Here's how the part is built. I have some questions about the finished solid (model axes, mm). Face numbers are marked on the shaded views. A direction names the side the tool comes from. Round coordinates to 2 decimals unless told otherwise and drop trailing zeros. Order: outer loops, then holes, each group sorted by start corner. A loop starts at its lowest first (then second) coordinate and runs counter-clockwise, first axis right, second up. Notation, with made-up numbers: (43, -20.75) -> (83, -20.75) arc R30 cw to (83, 17.25) -> close; hole circle Ø6 at (59, 23). An arc over 180 degrees is marked (long way). Use a Markdown table: item, result. Add a question column.
(1) I want a section at A-A, the plane y = 0. Please give me the cut outline in (x, z), then the cut area to 3 significant figures.
(2) If I drill on probe 1 along Y at (x, z) = (14.2, 9); probe 2 along Y at (x, z) = (0, 1); probe 3 along Y at (x, z) = (-5, 5.25), over which ranges is the centre line in solid material (lowest first)?
(3) I want a section at C-C, the plane z = 4.5. Please give me the cut outline in (x, y).
(4) Thinking about a two-plate mould opening in Y: for the marked faces 6, 7 and 8, which applies, pulls with the +Y half, pulls with the -Y half, needs draft (parallel to the pull), parting line crosses it, or undercut?
(5) On a 3-axis mill with a long thin cutter (end or side, diameter ignored), from which of +Z, -Z, +X, -X, +Y, -Y can I reach the whole of each face in a straight line? I mean the marked faces 1, 2, 3, 4 and 5. Say none if no direction works.
(6) I'm going to push flat-ended pins straight in: P1, Ø1.5, axis at x = -14.2, y = -14.2, coming from the +Z side; P2, Ø2, axis at x = -1.5, y = 12, coming from the -Z side; P3, Ø8, axis at x = 5.5, y = -3, coming from the +Z side. Where does each tip first touch, or does it pass through?
(7) I want a section at D-D, the plane y = -6. Please give me the cut outline in (x, z).
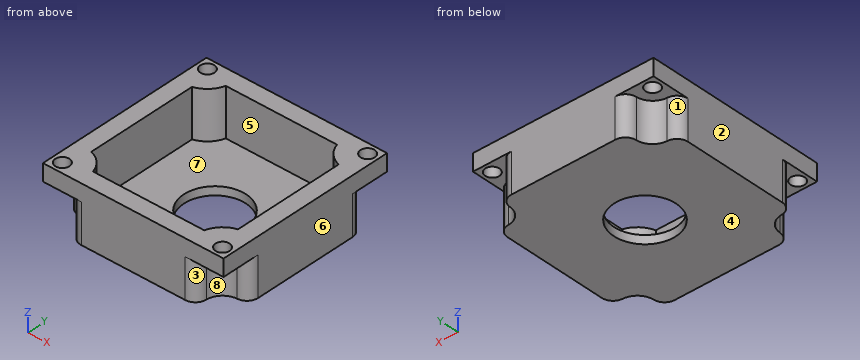
from build123d import *

# Parameters (mm, degrees)
SKETCH1_W           = 32
SKETCH1_H           = 32
SKETCH1_W_2         = 26
SKETCH1_H_2         = 26
BOSS_EXTRUDE1_DEPTH = 10
SKETCH2_W           = 26
SKETCH2_H           = 26
BOSS_EXTRUDE2_DEPTH = 1.5
SKETCH3_R           = 5.5
CUT_EXTRUDE1_DEPTH  = 9.5
SKETCH4_R           = 1.25
CUT_EXTRUDE2_DEPTH  = 21.5
SKETCH6_R           = 3
CUT_EXTRUDE3_DEPTH  = 7
SKETCH7_R           = 1.25
BOSS_EXTRUDE3_DEPTH = 3
CIRPATTERN1_COUNT   = 4
BOSS_EXTRUDE4_DEPTH = 8.5
CIRPATTERN2_COUNT   = 4
FILLET1_R           = 2


with BuildPart() as part:
    # Sketch1 → Boss-Extrude1 (new body)
    with BuildSketch(Plane.XY):
        Rectangle(SKETCH1_W, SKETCH1_H)
        Rectangle(SKETCH1_W_2, SKETCH1_H_2, mode=Mode.SUBTRACT)
    extrude(amount=BOSS_EXTRUDE1_DEPTH)

    # Sketch2 → Boss-Extrude2 (add)
    with BuildSketch(Plane(origin=(0, 0, 0), x_dir=(-1, 0, 0), z_dir=(0, 0, -1))):
        Rectangle(SKETCH2_W, SKETCH2_H)
    extrude(amount=-BOSS_EXTRUDE2_DEPTH)

    # Sketch3 → Cut-Extrude1 (cut)
    with BuildSketch(Plane(origin=(0, 0, 0), x_dir=(-1, 0, 0), z_dir=(0, 0, -1))):
        Circle(SKETCH3_R)
    extrude(amount=-CUT_EXTRUDE1_DEPTH, mode=Mode.SUBTRACT)

    # Sketch4 → Cut-Extrude2 (cut)
    with BuildSketch(Plane(origin=(0, 0, 0), x_dir=(-1, 0, 0), z_dir=(0, 0, -1))):
        with Locations((-14.2, 14.2)):
            Circle(SKETCH4_R)
        with Locations((14.2, 14.2)):
            Circle(SKETCH4_R)
        with Locations((14.2, -14.2)):
            Circle(SKETCH4_R)
        with Locations((-14.2, -14.2)):
            Circle(SKETCH4_R)
    extrude(amount=-CUT_EXTRUDE2_DEPTH, mode=Mode.SUBTRACT)

    # Sketch6 → Cut-Extrude3 (cut)
    with BuildSketch(Plane(origin=(0, 0, 0), x_dir=(-1, 0, 0), z_dir=(0, 0, -1))):
        with Locations((-14.2, 14.2)):
            Circle(SKETCH6_R)
        with Locations((14.2, 14.2)):
            Circle(SKETCH6_R)
        with Locations((14.2, -14.2)):
            Circle(SKETCH6_R)
        with Locations((-14.2, -14.2)):
            Circle(SKETCH6_R)
    extrude(amount=-CUT_EXTRUDE3_DEPTH, mode=Mode.SUBTRACT)

    # Sketch7 → Boss-Extrude3 (add)
    with BuildSketch(Plane(origin=(0, 0, 7), x_dir=(-1, 0, 0), z_dir=(0, 0, -1))):
        with BuildLine():
            ThreePointArc((11.8, 16), (11.220158645, 14.54719663), (11.450454583, 13))
            Line((11.450454583, 13), (13, 13))
            Line((13, 13), (13, 11.450454583))
            ThreePointArc((13, 11.450454583), (14.54719663, 11.220158645), (16, 11.8))
            Line((16, 11.8), (16, 16))
            Line((16, 16), (11.8, 16))
        make_face()
        with Locations((14.2, 14.2)):
            Circle(SKETCH7_R, mode=Mode.SUBTRACT)
        with BuildLine():
            Line((13, 13), (11.450454583, 13))
            ThreePointArc((11.450454583, 13), (12.078679656, 12.078679656), (13, 11.450454583))
            Line((13, 11.450454583), (13, 13))
        make_face()
    boss_extrude3 = extrude(amount=-BOSS_EXTRUDE3_DEPTH)

    # CirPattern1: Boss-Extrude3 ×4 about axis
    cirpattern1_axis = Axis((0, 0, 9.5), (0, 0, -1))
    for i in range(1, CIRPATTERN1_COUNT):
        add(boss_extrude3.rotate(cirpattern1_axis, i * 360 / CIRPATTERN1_COUNT))

    # Sketch8 → Boss-Extrude4 (add)
    with BuildSketch(Plane.XY.offset(1.5)):
        with BuildLine():
            ThreePointArc((-11.450454583, 13), (-12.078679656, 12.078679656), (-13, 11.450454583))
            Line((-13, 11.450454583), (-13, 9.862950312))
            ThreePointArc((-13, 9.862950312), (-11.018019485, 11.018019485), (-9.862950312, 13))
            Line((-9.862950312, 13), (-11.450454583, 13))
        make_face()
    boss_extrude4 = extrude(amount=BOSS_EXTRUDE4_DEPTH)

    # CirPattern2: Boss-Extrude4 ×4 about axis
    cirpattern2_axis = Axis((0, 0, 0), (0, 0, 1))
    for i in range(1, CIRPATTERN2_COUNT):
        add(boss_extrude4.rotate(cirpattern2_axis, i * 360 / CIRPATTERN2_COUNT))

    # Fillet1
    fillet1_edges = [part.edges().sort_by_distance(p)[0] for p in [
        (-16, -11.8, 3.5),
        (-11.8, -16, 3.5),
        (-16, 11.8, 3.5),
        (-11.8, 16, 3.5),
        (16, 11.8, 3.5),
        (11.8, 16, 3.5),
        (11.8, -16, 3.5),
        (16, -11.8, 3.5),
    ]]
    fillet(fillet1_edges, radius=FILLET1_R)


solid = part.part
Taken from the geometry:
| question | item | result |
|---|---|---|
| 1 | outline | (-16, 0) -> (-5.5, 0) -> (-5.5, 1.5) -> (-13, 1.5) -> (-13, 10) -> (-16, 10) -> close; (5.5, 0) -> (16, 0) -> (16, 10) -> (13, 10) -> (13, 1.5) -> (5.5, 1.5) -> close |
| 1 | area | 82.5 mm2 |
| 2 | probe 1 | y = -16 to -15.45, -12.95 to 12.95, 15.45 to 16 |
| 2 | probe 2 | y = -16 to -5.5, 5.5 to 16 |
| 2 | probe 3 | y = -16 to -13, 13 to 16 |
| 3 | outline | (-16, -9.2) arc R2 ccw to (-14.08, -11.2) arc R3 cw to (-11.2, -14.08) arc R2 ccw to (-9.2, -16) -> (9.2, -16) arc R2 ccw to (11.2, -14.08) arc R3 cw to (14.08, -11.2) arc R2 ccw to (16, -9.2) -> (16, 9.2) arc R2 ccw to (14.08, 11.2) arc R3 cw to (11.2, 14.08) arc R2 ccw to (9.2, 16) -> (-9.2, 16) arc R2 ccw to (-11.2, 14.08) arc R3 cw to (-14.08, 11.2) arc R2 ccw to (-16, 9.2) -> close; hole (-13, -9.86) arc R4.5 cw to (-9.86, -13) -> (9.86, -13) arc R4.5 cw to (13, -9.86) -> (13, 9.86) arc R4.5 cw to (9.86, 13) -> (-9.86, 13) arc R4.5 cw to (-13, 9.86) -> close |
| 4 | face 6 | needs draft |
| 4 | face 7 | undercut |
| 4 | face 8 | pulls with the -Y half |
| 5 | face 1 | -Z, -X, +Y |
| 5 | face 2 | +Z, -Z, -X, +Y, -Y |
| 5 | face 3 | -Z, +X, -Y |
| 5 | face 4 | -Z, +X, -X, +Y, -Y |
| 5 | face 5 | +Z |
| 6 | P1 | passes through |
| 6 | P2 | stops at z = 0 |
| 6 | P3 | stops at z = 1.5 |
| 7 | outline | (-16, 0) -> (16, 0) -> (16, 10) -> (13, 10) -> (13, 1.5) -> (-13, 1.5) -> (-13, 10) -> (-16, 10) -> close |
